Can you work these out from the model? Positions are in its coordinate system, mm. Round coordinates to 2 decimals unless told otherwise and drop trailing zeros. Loops run counter-clockwise (first coordinate to the right, second up) from the corner with the lowest first, then second, coordinate; pieces in that order, holes last. Notation, with made-up numbers: M 68,65 L 121,65 A12 cw 121,70 Z; hole C -26,51 d1. An arc over 180 degrees is marked long. Return JSON: item names as keys, results as strings.
```python
from build123d import *

# Parameters (mm, degrees)
SKETCH_1_W          = 10
SKETCH_1_H          = 3
EXTRUDE_1_DEPTH     = 395
SKETCH_2_W          = 4
SKETCH_2_H          = 3
CUT_EXTRUDE_1_DEPTH = 1168.363523234


with BuildPart() as part:
    # 草图1 → 凸台-拉伸1 (new body)
    with BuildSketch(Plane.XY.offset(1160.01)):
        with Locations((125.787596038, -4.889694097)):
            Rectangle(SKETCH_1_W, SKETCH_1_H)
    extrude(amount=-EXTRUDE_1_DEPTH)

    # 草图2 → 切除-拉伸1 (cut, through all)
    with BuildSketch(Plane(origin=(0, -3.389694097, 0), x_dir=(1, 0, 0), z_dir=(0, 1, 0))):
        with Locations((122.787596038, -891.51)):
            Rectangle(SKETCH_2_W, SKETCH_2_H)
        with Locations((122.787596038, -766.51)):
            Rectangle(SKETCH_2_W, SKETCH_2_H)
        with Locations((122.787596038, -1016.51)):
            Rectangle(SKETCH_2_W, SKETCH_2_H)
        with Locations((122.787596038, -1141.51)):
            Rectangle(SKETCH_2_W, SKETCH_2_H)
        with Locations((122.787596038, -1158.51)):
            Rectangle(SKETCH_2_W, SKETCH_2_H)
    extrude(amount=-CUT_EXTRUDE_1_DEPTH, mode=Mode.SUBTRACT)


solid = part.part
```
Q1. If I drill on line 1 along Z through (x, y) = (122.75, -5.05), over which ranges is the centre line in solid material (lowest first)?
Results:
{"line 1": "z = 768.01 to 890.01, 893.01 to 1015.01, 1018.01 to 1140.01, 1143.01 to 1157.01"}
Q2. I'm going to push flat-ended pins straight in: pin 1 Ø1.5 at (y, z) = (-4.5, 892) entering from -X; pin 2 Ø1.5 at (x, y) = (122.5, -4.5) entering from -Z; pin 3 Ø1.5 at (x, y) = (123.5, -5.5) entering from +Z. Where does each tip first touch, or does it pass through?
Results:
{"pin 1": "stops at x = 124.79", "pin 2": "stops at z = 768.01", "pin 3": "stops at z = 1157.01"}
Q3. Suppose I cut it at A-A, the plane y = -4.3. Please give me the cut outline in (x, z), plus the area to 3 significant figures.
Results:
{"outline": "M 120.79,768.01 L 124.79,768.01 L 124.79,765.01 L 130.79,765.01 L 130.79,1160.01 L 124.79,1160.01 L 124.79,1157.01 L 120.79,1157.01 L 120.79,1143.01 L 124.79,1143.01 L 124.79,1140.01 L 120.79,1140.01 L 120.79,1018.01 L 124.79,1018.01 L 124.79,1015.01 L 120.79,1015.01 L 120.79,893.01 L 124.79,893.01 L 124.79,890.01 L 120.79,890.01 Z", "area": "3,890 mm2"}
